Input: dimensioned drawing with shaded views. Units: mm. Origin: part minimum x, y, z. A direction names the side the tool comes from. Coordinates: 2 decimals unless noted, no trailing zeros. Loops run counter-clockwise (first coordinate to the right, second up) from the corner with the lowest first, then second, coordinate; pieces in that order, holes last.
(1) Line query: L1, parallel to Y at x = 36, z = 4; L2, parallel to X at y = 22.5, z = 6. Output: solid intervals per line, ascending.
(2) Section A-A, the plane z = 2.5. Return loops of the section in (x, y), then the cut area to 3 significant figures.
(3) Mould query, pull axis Y, two halves, no side actions, for the marked faces 4, 5 and 6. Classes: released by +Y, released by -Y, zero draft, split by the parting line, or undercut.
(4) Contact query for flat-ended pins moving along their axis: P1, Ø1, axis at x = 12, z = 5, coming from the +Y side; P2, Ø2, axis at x = 29.5, z = 2.5, coming from the +Y side; P3, Ø2, axis at y = 36, z = 2.5, coming from the +X side. Output: stop coordinate, or through.
(5) Section B-B, the plane y = 27.5. Return loops of the section in (x, z).
(6) Set-up query: the marked faces 1, 2 and 3. Return all of +Z, -Z, +X, -X, +Y, -Y with unobstructed straight access to the full face (end or side cutting, diameter ignored); none if empty.
(7) Section D-D, the plane y = 13. Return loops of the section in (x, z), then the cut area to 3 significant figures.
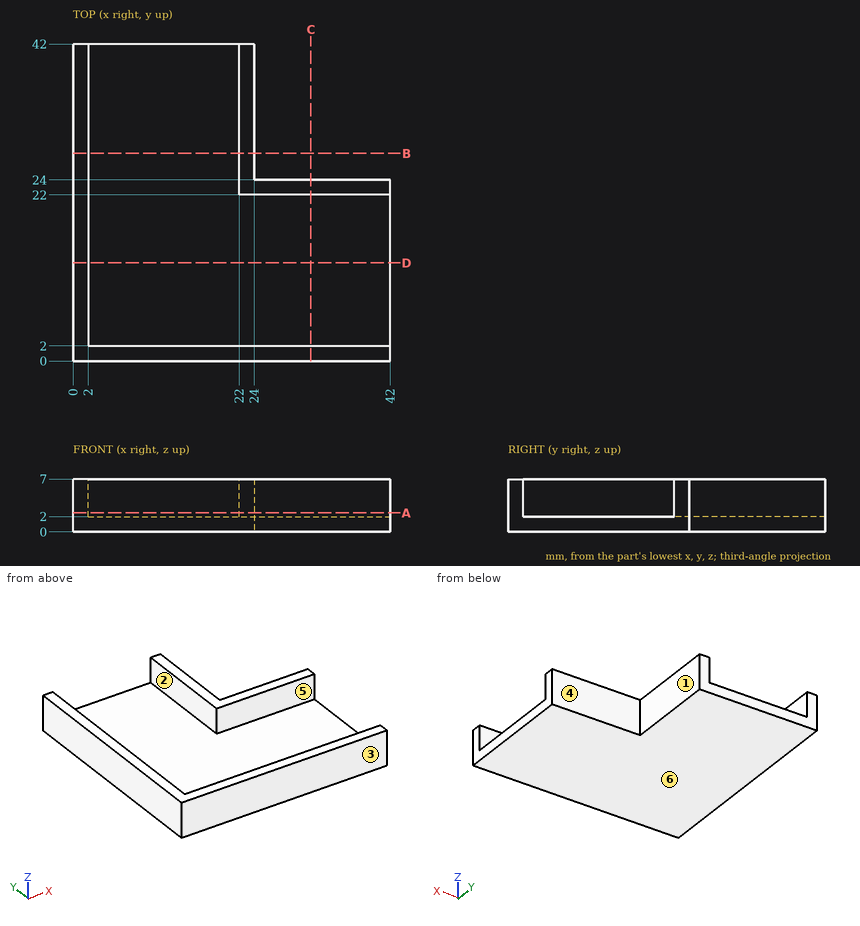
Report:
1. L1: y = 0 to 2, 22 to 24
1. L2: x = 0 to 2, 22 to 42
2. outline: (0, 0) - (42, 0) - (42, 2) - (2, 2) - (2, 42) - (0, 42) - close; (22, 22) - (42, 22) - (42, 24) - (24, 24) - (24, 42) - (22, 42) - close
2. area: 240 mm2
3. face 4: released by +Y
3. face 5: undercut
3. face 6: zero draft
4. P1: stops at y = 2
4. P2: stops at y = 24
4. P3: stops at x = 24
5. outline: (0, 0) - (24, 0) - (24, 7) - (22, 7) - (22, 2) - (2, 2) - (2, 7) - (0, 7) - close
6. face 1: +Z, -Z, +X, +Y
6. face 2: +Z, +Y
6. face 3: +Z, -Z, +X, -X, -Y
7. outline: (0, 0) - (42, 0) - (42, 2) - (2, 2) - (2, 7) - (0, 7) - close
7. area: 94.0 mm2
